Can you work these out from the model? Positions are in its coordinate system, mm. Face numbers are marked on the shaded views. Give positions to 0.01 mm unless a question says otherwise; leave off trailing zeros. Order: outer loops, then holes, each group sorted by start corner. A loop starts at its lowest first (then second) coordinate and runs counter-clockwise, first axis right, second up. Notation, with made-up numbers: (63.5, -8.5) -> (79.5, -8.5) arc R12 cw to (79.5, 13.5) -> close; hole circle Ø9 at (7.5, -0.5). An arc over 180 degrees is marked (long way). Answer as a JSON object with one key per item and string values.
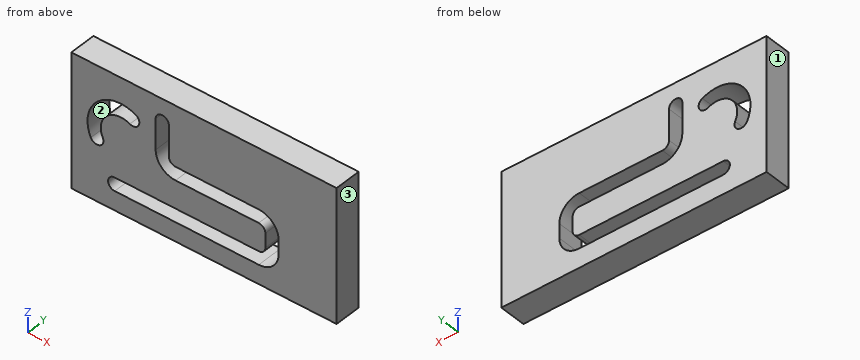
```python
from build123d import *

# Parameters (mm, degrees)
SKETCH1_W           = 254
SKETCH1_H           = 127
BOSS_EXTRUDE1_DEPTH = 25.4
CUT_EXTRUDE2_DEPTH  = 145.244271983
CUT_EXTRUDE3_DEPTH  = 145.244271983


with BuildPart() as part:
    # Sketch1 → Boss-Extrude1 (new body)
    with BuildSketch(Plane(origin=(0, 0, 0), x_dir=(1, 0, 0), z_dir=(0, 1, 0))):
        Rectangle(SKETCH1_W, SKETCH1_H)
    extrude(amount=BOSS_EXTRUDE1_DEPTH)

    # Sketch3 → Cut-Extrude2 (cut, through all)
    with BuildSketch(Plane(origin=(0, 25.4, 0), x_dir=(1, 0, 0), z_dir=(0, 1, 0))):
        with BuildLine():
            Line((-85.466243436, 32.694846332), (52.417137856, 32.694846332))
            ThreePointArc((52.417137856, 32.694846332), (56.907265917, 30.834974392), (58.767137856, 26.344846332))
            Line((58.767137856, 26.344846332), (58.767137856, 12.7))
            ThreePointArc((58.767137856, 12.7), (56.907265917, 8.209871939), (52.417137856, 6.35))
            Line((52.417137856, 6.35), (-27.235119701, 6.35))
            ThreePointArc((-27.235119701, 6.35), (-40.705503883, 0.770384182), (-46.285119701, -12.7))
            Line((-46.285119701, -12.7), (-46.285119701, -41.842848349))
            ThreePointArc((-46.285119701, -41.842848349), (-39.935119701, -48.192848349), (-33.585119701, -41.842848349))
            Line((-33.585119701, -41.842848349), (-33.585119701, -12.7))
            ThreePointArc((-33.585119701, -12.7), (-31.725247761, -8.209871939), (-27.235119701, -6.35))
            Line((-27.235119701, -6.35), (52.417137856, -6.35))
            ThreePointArc((52.417137856, -6.35), (65.887522038, -0.770384182), (71.467137856, 12.7))
            Line((71.467137856, 12.7), (71.467137856, 26.344846332))
            ThreePointArc((71.467137856, 26.344846332), (65.887522038, 39.815230513), (52.417137856, 45.394846332))
            Line((52.417137856, 45.394846332), (-85.466243436, 45.394846332))
            ThreePointArc((-85.466243436, 45.394846332), (-91.816243436, 39.044846332), (-85.466243436, 32.694846332))
        make_face()
    extrude(amount=-CUT_EXTRUDE2_DEPTH, mode=Mode.SUBTRACT)

    # Sketch4 → Cut-Extrude3 (cut, through all)
    with BuildSketch(Plane(origin=(0, 25.4, 0), x_dir=(1, 0, 0), z_dir=(0, 1, 0))):
        with BuildLine():
            ThreePointArc((-108.321717666, 6.889728777), (-102.153470481, -29.786963762), (-65.476777942, -35.955210947))
            ThreePointArc((-65.476777942, -35.955210947), (-62.539282648, -27.468979663), (-71.025513931, -24.531484369))
            ThreePointArc((-71.025513931, -24.531484369), (-93.17321436, -20.806707641), (-96.897991088, 1.340992788))
            ThreePointArc((-96.897991088, 1.340992788), (-99.835486382, 9.827224072), (-108.321717666, 6.889728777))
        make_face()
    extrude(amount=-CUT_EXTRUDE3_DEPTH, mode=Mode.SUBTRACT)


solid = part.part
```
1. If we section it at D-D on x = -83: Please give me the cut outline in (y, z), then the cut area to 3 significant figures.
Worked answers:
{"outline": "(0, -63.5) -> (25.4, -63.5) -> (25.4, -45.39) -> (0, -45.39) -> close; (0, -32.69) -> (25.4, -32.69) -> (25.4, 26.16) -> (0, 26.16) -> close; (0, 38.98) -> (25.4, 38.98) -> (25.4, 63.5) -> (0, 63.5) -> close", "area": "2,580 mm²"}
2. If we section it at C-C on z = -38.5: Please give me the cut outline in (x, y).
Worked answers:
{"outline": "(-127, 0) -> (-91.79, 0) -> (-91.79, 25.4) -> (-127, 25.4) -> close; (67.09, 0) -> (127, 0) -> (127, 25.4) -> (67.09, 25.4) -> close"}
3. Please list where these lines run through material, in increasing order: L1, parallel to Z at x = 43.5, y = 19; L2, parallel to Z at x = -79, y = 2.5; L3, parallel to X at y = 11.5, z = -17.5.
Worked answers:
{"L1": "-63.5 to -45.39, -32.69 to -6.35, 6.35 to 63.5", "L2": "-63.5 to -45.39, -32.69 to 26.47, 39.17 to 63.5", "L3": "-127 to 58.77, 71.47 to 127"}
4. If we mould it in two halves opening along X, with no side actions, what happens to the marked faces 1, 2 and 3? For each: +X half, -X half, draft (parallel to the pull), parting line (faces both ways), or undercut.
Worked answers:
{"face 1": "-X half", "face 2": "undercut", "face 3": "+X half"}
5. If we section it at B-B on y = 15: Please give me the cut outline in (x, z).
Worked answers:
{"outline": "(-127, -63.5) -> (127, -63.5) -> (127, 63.5) -> (-127, 63.5) -> close; hole (-108.32, -6.89) arc R6.35 ccw to (-96.9, -1.34) arc R19.36 cw to (-71.03, 24.53) arc R6.35 ccw to (-65.48, 35.96) arc R32.06 ccw to start; hole (-85.47, -45.39) -> (52.42, -45.39) arc R19.05 ccw to (71.47, -26.34) -> (71.47, -12.7) arc R19.05 ccw to (52.42, 6.35) -> (-27.24, 6.35) arc R6.35 cw to (-33.59, 12.7) -> (-33.59, 41.84) arc R6.35 ccw to (-46.29, 41.84) -> (-46.29, 12.7) arc R19.05 ccw to (-27.24, -6.35) -> (52.42, -6.35) arc R6.35 cw to (58.77, -12.7) -> (58.77, -26.34) arc R6.35 cw to (52.42, -32.69) -> (-85.47, -32.69) arc R6.35 ccw to start"}
6. If we section it at A-A on x = 50: Please give me the cut outline in (y, z), then the cut area to 3 significant figures.
Worked answers:
{"outline": "(0, -63.5) -> (25.4, -63.5) -> (25.4, -45.39) -> (0, -45.39) -> close; (0, -32.69) -> (25.4, -32.69) -> (25.4, -6.35) -> (0, -6.35) -> close; (0, 6.35) -> (25.4, 6.35) -> (25.4, 63.5) -> (0, 63.5) -> close", "area": "2,580 mm²"}
